from build123d import *

# Parameters (mm, degrees)
SKETCH_1_R          = 8
EXTRUDE_1_DEPTH     = 20
SKETCH_2_R          = 4
CUT_EXTRUDE_1_DEPTH = 13


with BuildPart() as part:
    # 草图1 → 凸台-拉伸1 (new body)
    with BuildSketch(Plane.XY):
        Circle(SKETCH_1_R)
    extrude(amount=EXTRUDE_1_DEPTH)

    # 草图2 → 切除-拉伸1 (cut)
    with BuildSketch(Plane.XY.offset(20)):
        Circle(SKETCH_2_R)
    extrude(amount=-CUT_EXTRUDE_1_DEPTH, mode=Mode.SUBTRACT)

    # 镜向1: part across plane


with BuildPart() as part_1:
    add(part.part)
    add(part.part.mirror(Plane.XY))


solid = part_1.part
Source: CAD feature listing. Evaluate the final solid. Frame: model axes, mm. A direction names the side the tool comes from. Give positions to 0.01 mm unless a question says otherwise; leave off trailing zeros. Write each loop counter-clockwise with the first axis right and the second up, starting at its lowest first coordinate (ties: lowest second). Pieces come first, ordered by that corner, then holes. Notation, with made-up numbers: (75, -16) -> (130, -16) arc R31 cw to (130, 23) -> close; hole circle Ø7 at (-13, 73.5). An arc over 180 degrees is marked (long way). Write item = value, one per line.
Q1. First-contact query: pin 1 (6.5 mm diameter, centred on x = 0, y = 0, fed in from -Z); pin 2 (8 mm diameter, centred on y = 5.5, z = 4, fed in from -X); pin 3 (4 mm diameter, centred on y = 3, z = 13, fed in from +X). Flat tips, straight axial feed; report the tip coordinate or a pass-through.
Here are the results:
pin_1 = -7
pin_2 = -7.86
pin_3 = 7.94
Q2. Cut plane C-C on z = -6. Return loops of the section in (x, y), then the cut area to 3 significant figures.
Here are the results:
outline = circle Ø16 at (0, 0)
area = 201 mm²
Q3. Cut plane A-A on y = 0. Return loops of the section in (x, z), then the cut area to 3 significant figures.
Here are the results:
outline = (-8, -20) -> (-4, -20) -> (-4, -7) -> (4, -7) -> (4, -20) -> (8, -20) -> (8, 20) -> (4, 20) -> (4, 7) -> (-4, 7) -> (-4, 20) -> (-8, 20) -> close
area = 432 mm²
Q4. Reachability of faces 4 (the face through (0, 0, 7)), 5 (the face through (0, 0, -7)), 6 (the face through (-4, -2, 20)) from +Z, -Z, +X, -X, +Y, -Y: full face, straight path, thin tool, end or side. Return the list, or none.
Here are the results:
face_4 = +Z
face_5 = -Z
face_6 = +Z, +X, -X, +Y, -Y
Q5. Cut plane D-D on z = -16. Return loops of the section in (x, y), then the cut area to 3 significant figures.
Here are the results:
outline = circle Ø16 at (0, 0); hole circle Ø8 at (0, 0)
area = 151 mm²
Q6. Line query: line 1 (Y direction, x = 0, z = 17); line 2 (X direction, y = -0.75, z = 10); line 3 (Y direction, x = 0.25, z = -2). Output: solid intervals per line, ascending. Write a range as from..to.
Here are the results:
line_1 = -8..-4, 4..8
line_2 = -7.96..-3.93, 3.93..7.96
line_3 = -8..8
Q7. Mould query, pull axis X, two halves, no side actions, for faces 1 (the face through (-4, -2, -20)), 2 (the face through (-0.867, -3.905, -13.591)), 3 (the face through (-1.73, -7.81, 0.28)). Classes: +X half, -X half, draft (parallel to the pull), parting line (faces both ways), or undercut.
Here are the results:
face_1 = draft
face_2 = undercut
face_3 = parting line
